The figure shows three views and two pictorial views of one solid part (mm, origin at its lowest corner). Answer the questions. Round coordinates to 2 decimals unless told otherwise and drop trailing zeros. Order: outer loops, then holes, each group sorted by start corner. A loop starts at its lowest first (then second) coordinate and runs counter-clockwise, first axis right, second up. Notation, with made-up numbers: (26.5, -34.75) - (73.5, -34.75) arc R15 ccw to (73.5, -14.75) - close; hole circle Ø7 at (-5.5, 21.25). An arc over 180 degrees is marked (long way). One line per item, written item: value. Start each with the question number.
1. Section C-C, the plane x = 101.74 is taken. Give the vertices of the cut face in (y, z) (3 decimals).
2. Section A-A, the plane y = 38.1 is taken. Give the vertices of the cut face in (x, z) (3 decimals), then the cut area to 3 significant figures.
3. Straight lines are drawn through the part: line 1 (Y direction, x = 101.74, z = 0.9); line 2 (Y direction, x = 75.5, z = 0.7); line 3 (X direction, y = 33, z = 0.4). For each, find the intervals that lie inside material, in ascending order.
4. A flat-ended cylindrical pin translates along its axis: P1, Ø8, axis at x = 34, y = 12.5, coming from the -Z side. Find the tip coordinate at first contact, or state that the pin passes through.
5. Section B-B, the plane z = 1.1 is taken. Give the vertices of the cut face in (x, y).
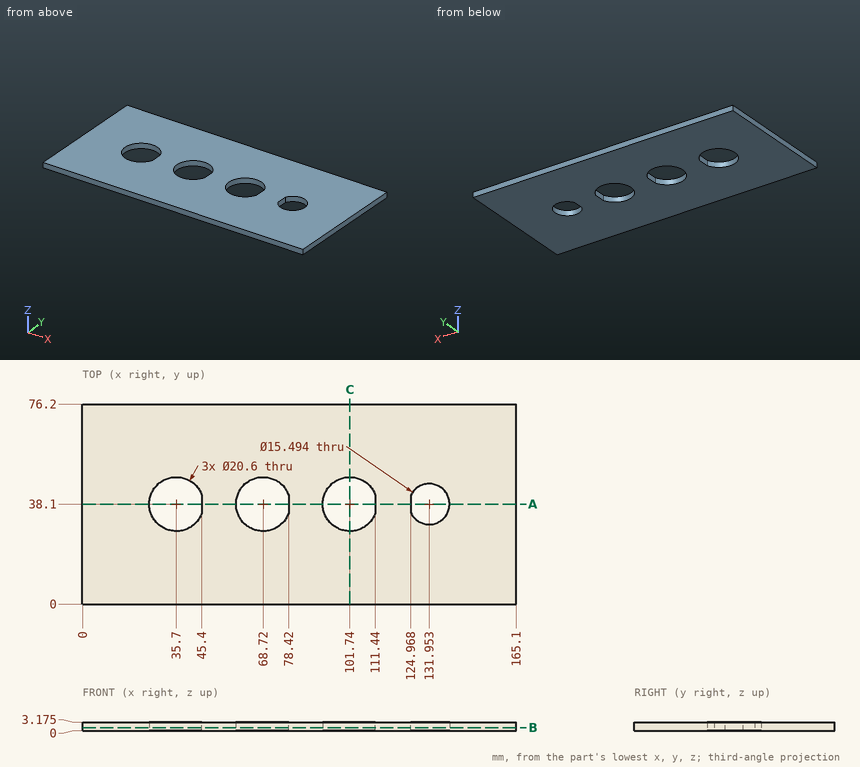
Answer list:
1. outline: (0, 0) - (27.8, 0) - (27.8, 3.175) - (0, 3.175) - close; (48.4, 0) - (76.2, 0) - (76.2, 3.175) - (48.4, 3.175) - close
2. outline: (0, 0) - (25.4, 0) - (25.4, 3.175) - (0, 3.175) - close; (45.4, 0) - (58.42, 0) - (58.42, 3.175) - (45.4, 3.175) - close; (78.42, 0) - (91.44, 0) - (91.44, 3.175) - (78.42, 3.175) - close; (111.44, 0) - (124.968, 0) - (124.968, 3.175) - (111.44, 3.175) - close; (139.7, 0) - (165.1, 0) - (165.1, 3.175) - (139.7, 3.175) - close
2. area: 287 mm²
3. line 1: y = 0 to 27.8, 48.4 to 76.2
3. line 2: y = 0 to 30.35, 45.85 to 76.2
3. line 3: x = 0 to 26.75, 44.65 to 59.77, 77.67 to 92.79, 110.69 to 126.12, 137.78 to 165.1
4. P1: stops at z = 0
5. outline: (0, 0) - (165.1, 0) - (165.1, 76.2) - (0, 76.2) - close; hole (45.4, 34.64) - (45.4, 41.56) arc R10.3 ccw (long way) to start; hole (78.42, 34.64) - (78.42, 41.56) arc R10.3 ccw (long way) to start; hole (111.44, 34.64) - (111.44, 41.56) arc R10.3 ccw (long way) to start; hole (124.97, 34.75) arc R7.75 ccw (long way) to (124.97, 41.45) - close
